Here's how the part is built. I have some questions about the finished solid (model axes, mm). A direction names the side the tool comes from. Give positions to 0.01 mm unless a question says otherwise; leave off trailing zeros. Write each loop counter-clockwise with the first axis right and the second up, starting at its lowest first coordinate (ties: lowest second). Pieces come first, ordered by that corner, then holes. Notation, with made-up numbers: (75.5, 49.25) - (111.5, 49.25) arc R18 ccw to (111.5, 84.25) - close; hole circle Ø4 at (56.25, 88). An arc over 180 degrees is marked (long way). One line per item, written item: value. Start each with the question number.
1) On a 3-axis mill with a long thin cutter (end or side, diameter ignored), from which of +Z, -Z, +X, -X, +Y, -Y can I reach the whole of each face in a straight line? I mean faces 1 (the flat face through (-8, -148, -12.5)), 2 (the flat face through (-6.912, -147.9, 5.406)), 3 (the flat face through (-12.5, -148, -8)), 4 (the flat face through (-4.38, -148, 0)), 5 (the flat face through (0, -148, -4.38)). Say none if no direction works.
2) We'd pull the mould along X, two halves only. Please class faces 6 (the flat face through (12.5, -148, 8)), 7 (the flat face through (0, -148, 4.38)), 8 (the flat face through (6.848, -147.9, 5.342)), 9 (the flat face through (0, -300, 3)): +X half, -X half, draft (parallel to the pull), parting line (faces both ways), or undercut.
3) I'm going to push flat-ended pins straight in: P1, Ø2, axis at x = -3, y = -89.5, coming from the +Z side; P2, Ø2, axis at y = -61.5, z = 1.5, coming from the +X side; P3, Ø2.5, axis at x = 1, y = -180.5, coming from the +Z side. Where does each tip first touch, or does it pass through?
4) Imagine slicing it at B-B on z = 0. Write out the boundary of the cut face in (x, y), plus the area to 3 significant figures.
5) Imagine slicing it at A-A on x = 0. Write out the boundary of the cut face in (y, z).
6) Please list where these lines run through material, in increasing order: L1, parallel to Z at x = 0, y = -185.5; L2, parallel to Z at x = 9.5, y = -93.5; L3, parallel to Z at x = 5, y = -185.5. Write a range as [from, to].
from build123d import *

# Parameters (mm, degrees)
F0_R     = 2.5
F1_DEPTH = 300


# Not quite as in the source:
# - ends of sketch curves that miss each other by under 0.0002 mm in the source are joined


with BuildPart() as f1:
    # F0 (on Front) → F1 (new body)
    with BuildSketch(Plane.XZ):
        with BuildLine():
            ThreePointArc((12.5, 11.8), (12.2949747468, 12.2949747468), (11.8, 12.5))
            Line((11.8, 12.5), (4.3149960966, 12.5))
            ThreePointArc((4.3149960966, 12.5), (3.5629475094, 12.1890874766), (3.25, 11.4378834224))
            Line((3.25, 11.4378834224), (3.2499960966, 11.4350005532))
            ThreePointArc((3.2499960966, 11.4350005532), (3.5619271791, 10.6819314736), (4.3149960966, 10.37))
            Line((4.3149960966, 10.37), (7.1739130624, 10.37))
            ThreePointArc((7.1739130624, 10.37), (7.8206287352, 9.9378784027), (7.6688878092, 9.1750252532))
            Line((7.6688878092, 9.1750252532), (3.0788878092, 4.5850252532))
            ThreePointArc((3.0788878092, 4.5850252532), (2.8517914651, 4.4332843272), (2.5839130624, 4.38))
            Line((2.5839130624, 4.38), (-2.5839130624, 4.38))
            ThreePointArc((-2.5839130624, 4.38), (-2.8517914651, 4.4332843272), (-3.0788878092, 4.5850252532))
            Line((-3.0788878092, 4.5850252532), (-7.6688878092, 9.1750252532))
            ThreePointArc((-7.6688878092, 9.1750252532), (-7.8206287352, 9.9378784027), (-7.1739130624, 10.37))
            Line((-7.1739130624, 10.37), (-4.3149983424, 10.37))
            ThreePointArc((-4.3149983424, 10.37), (-3.2499983424, 11.435), (-4.3149983424, 12.5))
            Line((-4.3149983424, 12.5), (-11.8, 12.5))
            ThreePointArc((-11.8, 12.5), (-12.2949747468, 12.2949747468), (-12.5, 11.8))
            Line((-12.5, 11.8), (-12.5, 4.3148727296))
            ThreePointArc((-12.5, 4.3148727296), (-11.435, 3.2498727296), (-10.37, 4.3148727296))
            Line((-10.37, 4.3148727296), (-10.37, 7.1739130624))
            ThreePointArc((-10.37, 7.1739130624), (-9.9378784027, 7.8206287352), (-9.1750252532, 7.6688878092))
            Line((-9.1750252532, 7.6688878092), (-4.5850252532, 3.0788878092))
            ThreePointArc((-4.5850252532, 3.0788878092), (-4.4332843272, 2.8517914651), (-4.38, 2.5839130624))
            Line((-4.38, 2.5839130624), (-4.38, -2.5839130624))
            ThreePointArc((-4.38, -2.5839130624), (-4.4332843272, -2.8517914651), (-4.5850252532, -3.0788878092))
            Line((-4.5850252532, -3.0788878092), (-9.1750252532, -7.6688878092))
            ThreePointArc((-9.1750252532, -7.6688878092), (-9.9378784027, -7.8206287352), (-10.37, -7.1739130624))
            Line((-10.37, -7.1739130624), (-10.37, -4.3142225218))
            ThreePointArc((-10.37, -4.3142225218), (-11.435, -3.2492225218), (-12.5, -4.3142225218))
            Line((-12.5, -4.3142225218), (-12.5, -11.8))
            ThreePointArc((-12.5, -11.8), (-12.2949747468, -12.2949747468), (-11.8, -12.5))
            Line((-11.8, -12.5), (-4.3149983424, -12.5))
            ThreePointArc((-4.3149983424, -12.5), (-3.2499983424, -11.435), (-4.3149983424, -10.37))
            Line((-4.3149983424, -10.37), (-7.1739130624, -10.37))
            ThreePointArc((-7.1739130624, -10.37), (-7.8206287352, -9.9378784027), (-7.6688878092, -9.1750252532))
            Line((-7.6688878092, -9.1750252532), (-3.0788878092, -4.5850252532))
            ThreePointArc((-3.0788878092, -4.5850252532), (-2.8517914651, -4.4332843272), (-2.5839130624, -4.38))
            Line((-2.5839130624, -4.38), (2.5839130624, -4.38))
            ThreePointArc((2.5839130624, -4.38), (2.8517914651, -4.4332843272), (3.0788878092, -4.5850252532))
            Line((3.0788878092, -4.5850252532), (7.6688878092, -9.1750252532))
            ThreePointArc((7.6688878092, -9.1750252532), (7.8206287352, -9.9378784027), (7.1739130624, -10.37))
            Line((7.1739130624, -10.37), (4.3149960966, -10.37))
            ThreePointArc((4.3149960966, -10.37), (3.2499960966, -11.435), (4.3149960966, -12.5))
            Line((4.3149960966, -12.5), (11.8, -12.5))
            ThreePointArc((11.8, -12.5), (12.2949747468, -12.2949747468), (12.5, -11.8))
            Line((12.5, -11.8), (12.5, -4.3148727296))
            Line((12.5, -4.3148727296), (12.5, -4.3142225218))
            ThreePointArc((12.5, -4.3142225218), (11.435, -3.2498727296), (10.3700001985, -4.314222522))
            Line((10.3700001985, -4.314222522), (10.37, -4.3148727296))
            Line((10.37, -4.3148727296), (10.37, -7.1739130624))
            ThreePointArc((10.37, -7.1739130624), (9.9378784027, -7.8206287352), (9.1750252532, -7.6688878092))
            Line((9.1750252532, -7.6688878092), (4.5850252532, -3.0788878092))
            ThreePointArc((4.5850252532, -3.0788878092), (4.4332843272, -2.8517914651), (4.38, -2.5839130624))
            Line((4.38, -2.5839130624), (4.38, 2.5839130624))
            ThreePointArc((4.38, 2.5839130624), (4.4332843272, 2.8517914651), (4.5850252532, 3.0788878092))
            Line((4.5850252532, 3.0788878092), (9.1750252532, 7.6688878092))
            ThreePointArc((9.1750252532, 7.6688878092), (9.9378784027, 7.8206287352), (10.37, 7.1739130624))
            Line((10.37, 7.1739130624), (10.37, 4.3148727296))
            ThreePointArc((10.37, 4.3148727296), (10.3700000496, 4.3145476258), (10.3700001985, 4.314222522))
            ThreePointArc((10.3700001985, 4.314222522), (11.435, 3.2498727296), (12.4999998015, 4.314222522))
            ThreePointArc((12.4999998015, 4.314222522), (12.4999999504, 4.3145476258), (12.5, 4.3148727296))
            Line((12.5, 4.3148727296), (12.5, 11.8))
        make_face()
        Circle(F0_R, mode=Mode.SUBTRACT)
        with BuildLine():
            ThreePointArc((10.37, 4.3142225218), (11.435, 3.2492225218), (12.5, 4.3142225218))
            ThreePointArc((12.5, 4.3142225218), (11.435, 3.2498727296), (10.37, 4.3142225218))
        make_face()
        with BuildLine():
            ThreePointArc((12.5, -4.3142225218), (11.435, -3.2492225218), (10.37, -4.3142225218))
            ThreePointArc((10.37, -4.3142225218), (11.435, -3.2498727296), (12.5, -4.3142225218))
        make_face()
    extrude(amount=F1_DEPTH)


solid = f1.part
Numbers:
1. face 1: -Z, +X, -X, +Y, -Y
1. face 2: +Y, -Y
1. face 3: +Z, -Z, -X, +Y, -Y
1. face 4: -X, +Y, -Y
1. face 5: -Z, +Y, -Y
2. face 6: +X half
2. face 7: undercut
2. face 8: undercut
2. face 9: draft
3. P1: z = 12.45
3. P2: x = 4.38
3. P3: z = 4.38
4. outline: (-4.38, -300) - (-2.5, -300) - (-2.5, 0) - (-4.38, 0) - close; (2.5, -300) - (4.38, -300) - (4.38, 0) - (2.5, 0) - close
4. area: 1,130 mm^2
5. outline: (-300, -4.38) - (0, -4.38) - (0, -2.5) - (-300, -2.5) - close; (-300, 2.5) - (0, 2.5) - (0, 4.38) - (-300, 4.38) - close
6. L1: [-4.38, -2.5], [2.5, 4.38]
6. L2: [-12.5, -7.85], [7.85, 12.5]
6. L3: [-12.5, -10.37], [-6.51, -3.49], [3.49, 6.51], [10.37, 12.5]
